Here's the drawing with two shaded views (mm, measured from the low corner). I have some questions. Coordinates: 2 decimals unless noted, no trailing zeros. Loops run counter-clockwise (first coordinate to the right, second up) from the corner with the lowest first, then second, coordinate; pieces in that order, holes last. Notation, with made-up numbers: (40, -27.5) -> (52, -27.5) arc R9 cw to (52, -11.5) -> close; hole circle Ø7 at (2, 42.5). An arc over 180 degrees is marked (long way). Answer as a JSON object with one key per item and string values. Group by question number.
1) I want a section at D-D (x = 74). Write out the boundary of the cut face in (y, z).
2) I want a section at B-B (x = 24). Write out the boundary of the cut face in (y, z).
3) I want a section at A-A (y = 40). Write out the boundary of the cut face in (x, z), then the cut area to 3 significant figures.
4) I'm going to push flat-ended pins straight in: pin 1 (3 mm diameter, centred on y = 53, z = 105, fed in from +X); pin 2 (1 mm diameter, centred on x = 43, z = 26, fed in from -Y); pin 3 (11 mm diameter, centred on x = 23.5, y = 49, fed in from -Z). Where does each tip first touch, or does it pass through?
5) I need wall thicknesses on probe 1 along X at (y, z) = (42, 106.5); probe 2 along Z at (x, y) = (110.5, 44); probe 3 along Y at (x, z) = (71, 33.5). Which ranges of each line are inside material? Lowest first, please. Write a range as [from, to].
6) I want a section at C-C (z = 22.5). Write out the boundary of the cut face in (x, y), then the cut area to 3 significant figures.
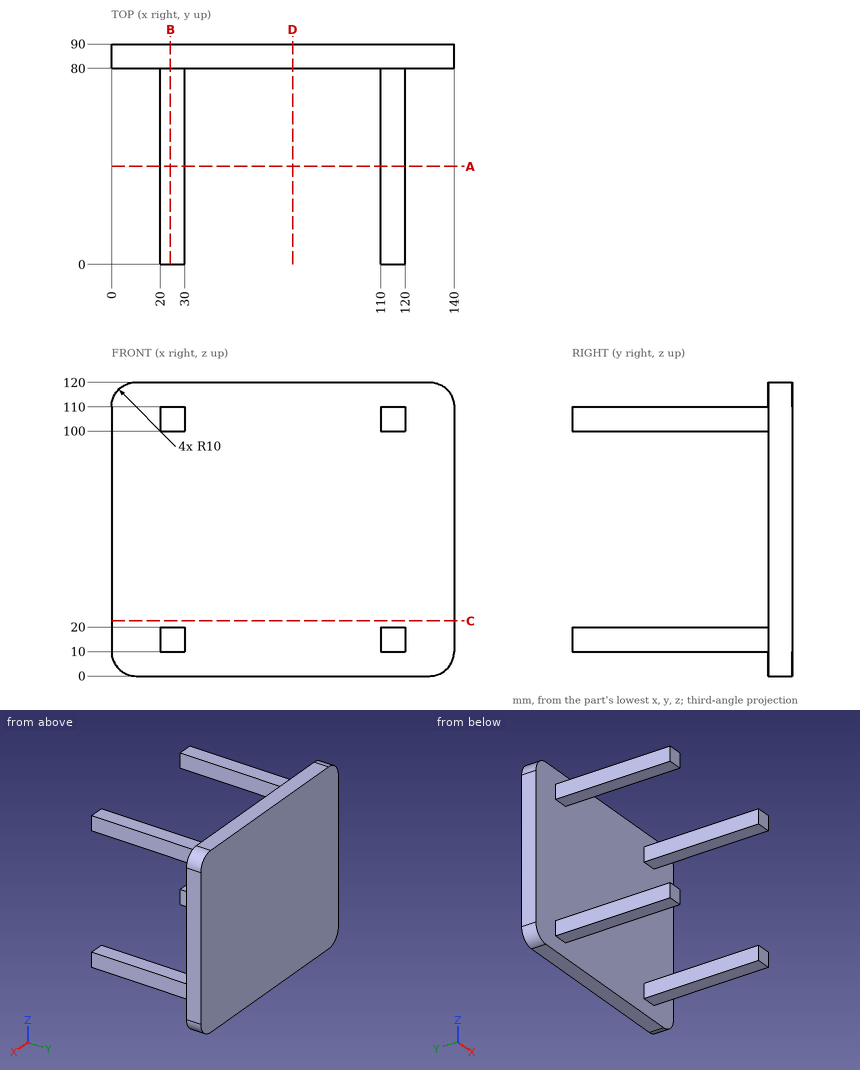
Determined:
{
 "1": {"outline": "(80, 0) -> (90, 0) -> (90, 120) -> (80, 120) -> close"},
 "2": {"outline": "(0, 10) -> (80, 10) -> (80, 0) -> (90, 0) -> (90, 120) -> (80, 120) -> (80, 110) -> (0, 110) -> (0, 100) -> (80, 100) -> (80, 20) -> (0, 20) -> close"},
 "3": {"outline": "(20, 10) -> (30, 10) -> (30, 20) -> (20, 20) -> close; (20, 100) -> (30, 100) -> (30, 110) -> (20, 110) -> close; (110, 10) -> (120, 10) -> (120, 20) -> (110, 20) -> close; (110, 100) -> (120, 100) -> (120, 110) -> (110, 110) -> close", "area": "400 mm^2"},
 "4": {"pin 1": "x = 120", "pin 2": "y = 80", "pin 3": "z = 10"},
 "5": {"probe 1": "[20, 30], [110, 120]", "probe 2": "[10, 20], [100, 110]", "probe 3": "[80, 90]"},
 "6": {"outline": "(0, 80) -> (140, 80) -> (140, 90) -> (0, 90) -> close", "area": "1,400 mm^2"}
}
